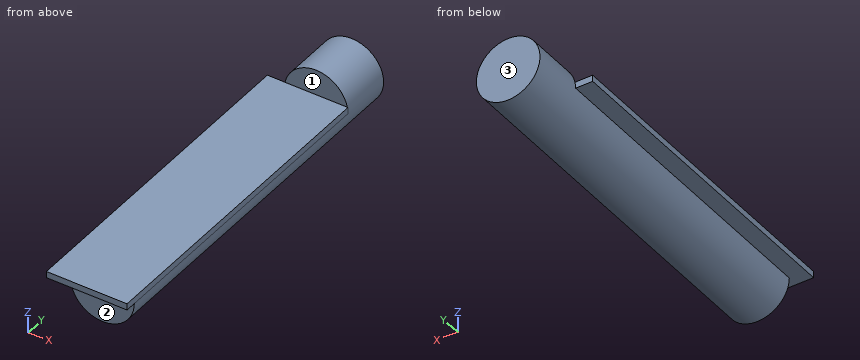
```python
from build123d import *

# Parameters (mm, degrees)
F1_DEPTH = 150
F3_R     = 15
F4_DEPTH = 25
F5_W     = 38.047614
F5_H     = 3
F6_DEPTH = 155.1


with BuildPart() as f1:
    # F0 (on Front) → F1 (new body)
    with BuildSketch(Plane.XZ):
        with BuildLine():
            Line((15, 0), (-15, 0))
            ThreePointArc((-15, 0), (0, -15), (15, 0))
        make_face()
    extrude(amount=F1_DEPTH)

    # F3 (on Front) → F4 (join)
    with BuildSketch(Plane.XZ):
        Circle(F3_R)
    extrude(amount=-F4_DEPTH)

    # F5 (on face) → F6 (join)
    with BuildSketch(Plane.XZ):
        with Locations((-4.023807, 1.5)):
            Rectangle(F5_W, F5_H)
    extrude(amount=F6_DEPTH)


solid = f1.part
```
The listing builds one solid part. Answer for the finished solid, in the listing's coordinates (mm). Face numbers are marked on the shaded views. A direction names the side the tool comes from. Give positions to 0.01 mm unless a question says otherwise; leave off trailing zeros. Loops run counter-clockwise (first coordinate to the right, second up) from the corner with the lowest first, then second, coordinate; pieces in that order, holes last. Notation, with made-up numbers: M -32.5,87.5 L 2.5,87.5 A20 cw 2.5,91.5 Z; hole C -2.5,-20 d3. An arc over 180 degrees is marked long. One line per item, written item: value.
Q1. A cutting plane is placed at C-C on y = -98. Determine the outline of the cut face in (x, z).
Working result:
outline: M -23.05,0 L -15,0 A15 ccw 15,0 L 15,3 L -23.05,3 Z
Q2. A cutting plane is placed at B-B on z = 1.5. Determine the outline of the cut face in (x, y), then the cut area to 3 significant figures.
Working result:
outline: M -23.05,-155.1 L 15,-155.1 L 15,0 L 14.92,0 L 14.92,25 L -14.92,25 L -14.92,0 L -23.05,0 Z
area: 6,650 mm^2
Q3. A cutting plane is placed at A-A on x = 0. Determine the outline of the cut face in (y, z).
Working result:
outline: M -155.1,0 L -150,0 L -150,-15 L 25,-15 L 25,15 L 0,15 L 0,3 L -155.1,3 Z
Q4. Find the intervals of material crossed by line 1 (Z direction, x = -1, y = -13.5); line 2 (Y direction, x = -13, z = -0.5); line 3 (Y direction, x = 6.5, z = 12), in increasing order. Write a range as from..to.
Working result:
line 1: z = -14.97..3
line 2: y = -150..25
line 3: y = 0..25
Q5. Flat-ended cylindrical pins translate along their axes: P1, Ø19, axis at x = 2, y = -79, coming from the +Z side; P2, Ø6, axis at x = -1, z = 8.5, coming from the -Y side; P3, Ø6, axis at y = -134.5, z = -4.5, coming from the +X side. Find the tip coordinate at first contact, or state that the pin passes through.
Working result:
P1: stops at z = 3
P2: stops at y = 0
P3: stops at x = 14.92
Q6. A cutting plane is placed at D-D on z = -10.5. Determine the outline of the cut face in (x, y), then the cut area to 3 significant figures.
Working result:
outline: M -10.71,-150 L 10.71,-150 L 10.71,25 L -10.71,25 Z
area: 3,750 mm^2
Q7. For the marked faces 1, 2 and 3, determine the directions among +Z, -Z, +X, -X, +Y, -Y from which every point of the face is accessible in a straight line to the end or side of a thin tool.
Working result:
face 1: +Z, +X, -X, -Y
face 2: -Z, +X, -X, -Y
face 3: +Z, -Z, +X, -X, +Y
